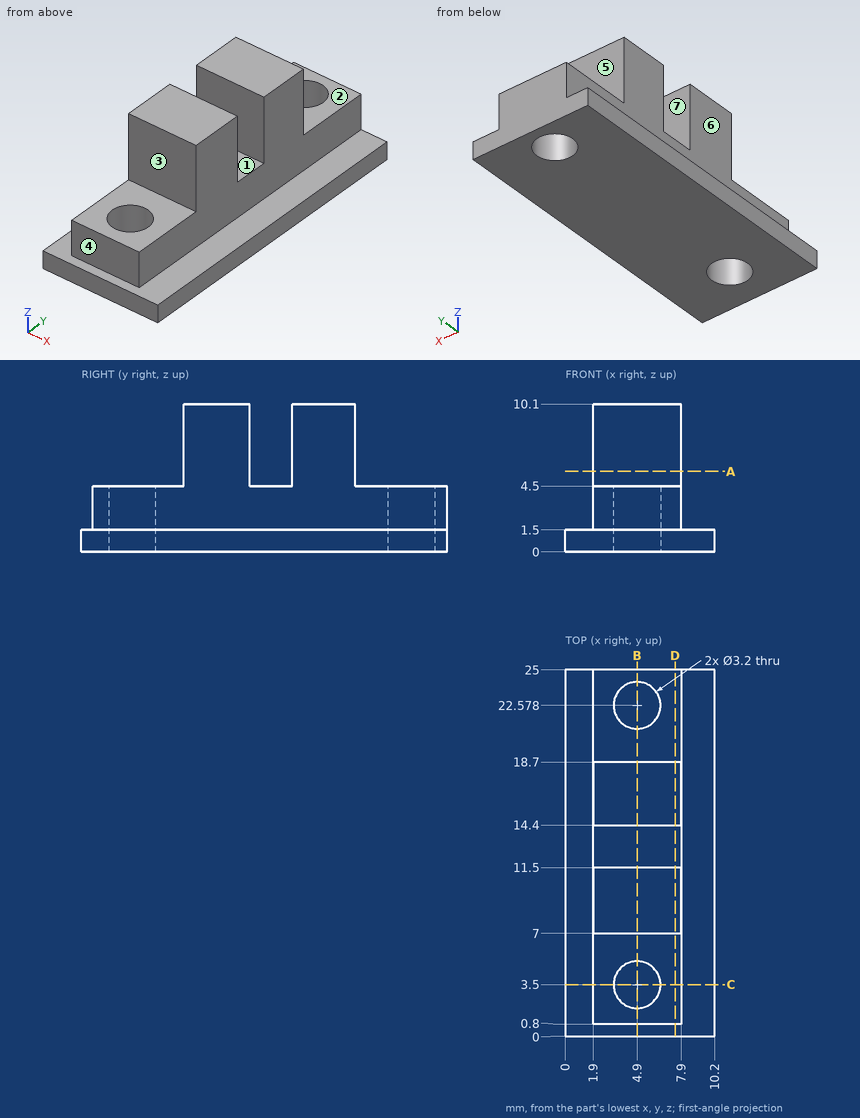
For this review, use the dimensioned drawing (mm, ordinates from the lowest corner) and the shaded views. A direction names the side the tool comes from. Coordinates: 2 decimals unless noted, no trailing zeros. Loops run counter-clockwise (first coordinate to the right, second up) from the corner with the lowest first, then second, coordinate; pieces in that order, holes last.
1. Mouldability with a two-part tool opening along Y and no side actions: class the marked faces 1, 2 and 3 as +Y half, -Y half, draft (parallel to the pull), parting line (faces both ways), or undercut.
2. Insertion check: P1, Ø2.5, axis at x = 4.9, y = 22.58, coming from the -Z side; P2, Ø3, axis at x = 5.5, z = 8, coming from the +Y side; P3, Ø6, axis at x = 6, z = 8, coming from the -Y side; P4, Ø4.5, axis at y = 13, z = 4.5, coming from the -X side. Each pin has a flat end and moves straight along its axis. Give the tip position at first contact, or say it passes through.
3. Add section B-B, the plane x = 4.9. Give the boundary of the cut face in (y, z), then the cut area to 3 significant figures.
4. For the marked faces 4, 5, 6 and 7, list the 3-axis set-ups (+Z, -Z, +X, -X, +Y, -Y) from which the entire face can be reached by the end or side of a thin tool; tool diameter is ignored.
5. For line 1 (Y direction, x = 4.9, z = 1.55); line 2 (Y direction, x = 6.75, z = 4.75); line 3 (X direction, y = 14, z = 2.25), list the stretches that pass through material, from the lowest coordinate up.
6. Add section A-A, the plane z = 5.5. Give the boundary of the cut face in (x, y).
7. Add section C-C, the plane y = 3.5. Give the boundary of the cut face in (x, z), then the cut area to 3 significant figures.
8. Add section D-D, the plane x = 7.5. Give the boundary of the cut face in (y, z), then the cut area to 3 significant figures.
Result:
1. face 1: undercut
1. face 2: draft
1. face 3: -Y half
2. P1: passes through
2. P2: stops at y = 18.7
2. P3: stops at y = 7
2. P4: stops at x = 1.9
3. outline: (0, 0) - (1.9, 0) - (1.9, 4.5) - (0.8, 4.5) - (0.8, 1.5) - (0, 1.5) - close; (5.1, 0) - (20.98, 0) - (20.98, 4.5) - (18.7, 4.5) - (18.7, 10.1) - (14.4, 10.1) - (14.4, 4.5) - (11.5, 4.5) - (11.5, 10.1) - (7, 10.1) - (7, 4.5) - (5.1, 4.5) - close; (24.18, 0) - (25, 0) - (25, 4.5) - (24.18, 4.5) - close
3. area: 131 mm2
4. face 4: +Z, +X, -X, -Y
4. face 5: +Z, +X, -X, +Y
4. face 6: +Z, -X, +Y, -Y
4. face 7: +Z, +X, -X
5. line 1: y = 0.8 to 1.9, 5.1 to 20.98, 24.18 to 25
5. line 2: y = 7 to 11.5, 14.4 to 18.7
5. line 3: x = 1.9 to 7.9
6. outline: (1.9, 7) - (7.9, 7) - (7.9, 11.5) - (1.9, 11.5) - close; (1.9, 14.4) - (7.9, 14.4) - (7.9, 18.7) - (1.9, 18.7) - close
7. outline: (0, 0) - (3.3, 0) - (3.3, 4.5) - (1.9, 4.5) - (1.9, 1.5) - (0, 1.5) - close; (6.5, 0) - (10.2, 0) - (10.2, 1.5) - (7.9, 1.5) - (7.9, 4.5) - (6.5, 4.5) - close
7. area: 18.9 mm2
8. outline: (0, 0) - (25, 0) - (25, 4.5) - (18.7, 4.5) - (18.7, 10.1) - (14.4, 10.1) - (14.4, 4.5) - (11.5, 4.5) - (11.5, 10.1) - (7, 10.1) - (7, 4.5) - (0.8, 4.5) - (0.8, 1.5) - (0, 1.5) - close
8. area: 159 mm2
